```python
from build123d import *

# Parameters (mm, degrees)
SKETCH1_W           = 23
SKETCH1_H           = 13
BOSS_EXTRUDE1_DEPTH = 18
SKETCH2_W           = 33
SKETCH2_H           = 13
BOSS_EXTRUDE2_DEPTH = 2.5
SKETCH3_W           = 23
SKETCH3_H           = 13
BOSS_EXTRUDE3_DEPTH = 1.5
BOSS_EXTRUDE4_DEPTH = 5.5
SKETCH5_R           = 2.4
BOSS_EXTRUDE5_DEPTH = 4


with BuildPart() as part:
    # Sketch1 → Boss-Extrude1 (new body)
    with BuildSketch(Plane(origin=(0, 0, 0), x_dir=(1, 0, 0), z_dir=(0, 1, 0))):
        Rectangle(SKETCH1_W, SKETCH1_H)
    extrude(amount=BOSS_EXTRUDE1_DEPTH)

    # Sketch2 → Boss-Extrude2 (add)
    with BuildSketch(Plane(origin=(0, 18, 0), x_dir=(1, 0, 0), z_dir=(0, 1, 0))):
        Rectangle(SKETCH2_W, SKETCH2_H)
    extrude(amount=BOSS_EXTRUDE2_DEPTH)

    # Sketch3 → Boss-Extrude3 (add)
    with BuildSketch(Plane(origin=(0, 20.5, 0), x_dir=(1, 0, 0), z_dir=(0, 1, 0))):
        Rectangle(SKETCH3_W, SKETCH3_H)
    extrude(amount=BOSS_EXTRUDE3_DEPTH)

    # Sketch4 → Boss-Extrude4 (add)
    with BuildSketch(Plane(origin=(0, 22, 0), x_dir=(1, 0, 0), z_dir=(0, 1, 0))):
        with BuildLine():
            ThreePointArc((0.918269231, 2.687766603), (-11.5, 0), (0.918269231, -2.687766603))
            ThreePointArc((0.918269231, -2.687766603), (4.25, 0), (0.918269231, 2.687766603))
        make_face()
    extrude(amount=BOSS_EXTRUDE4_DEPTH)

    # Sketch5 → Boss-Extrude5 (add)
    with BuildSketch(Plane(origin=(0, 27.5, 0), x_dir=(1, 0, 0), z_dir=(0, 1, 0))):
        with Locations(Location((-5, 0, 0), (0, 0, 270))):
            Circle(SKETCH5_R)
    extrude(amount=BOSS_EXTRUDE5_DEPTH)


solid = part.part
```
Verification items for the finished model (mm, model axes). A direction names the side the tool comes from. Coordinates: 2 decimals unless noted, no trailing zeros. Loops run counter-clockwise (first coordinate to the right, second up) from the corner with the lowest first, then second, coordinate; pieces in that order, holes last. Notation, with made-up numbers: (34.5, 57) - (51.5, 57) arc R15 ccw to (51.5, 72) - close; hole circle Ø11 at (63, 60). An arc over 180 degrees is marked (long way). Put each result on its own line as item: value.
Item 1: Section check D-D (x = 14). Enter the section's corners in (y, z).
Conclusion:
outline: (18, -6.5) - (20.5, -6.5) - (20.5, 6.5) - (18, 6.5) - close
Item 2: Section check B-B (z = -4.5). Enter the section's corners in (x, y), then the cut area to 3 significant figures.
Conclusion:
outline: (-16.5, 18) - (-11.5, 18) - (-11.5, 0) - (11.5, 0) - (11.5, 18) - (16.5, 18) - (16.5, 20.5) - (11.5, 20.5) - (11.5, 22) - (-0.31, 22) - (-0.31, 27.5) - (-9.69, 27.5) - (-9.69, 22) - (-11.5, 22) - (-11.5, 20.5) - (-16.5, 20.5) - close
area: 583 mm2
Item 3: Set-up check for faces 1 (the face through (11.5, 21, 0)), 2 (the face through (14, 18, 0)), 3 (the face through (-2.976, 29.472, 1.29)): record each of +Z, -Z, +X, -X, +Y, -Y from which the full face is reachable in a straight line by a thin tool's end or side.
Conclusion:
face 1: +Z, -Z, +X, +Y
face 2: +Z, -Z, +X, -Y
face 3: +Y
Item 4: Gauge pin test, flat ends, axial feed: pin 1 Ø1.5 at (x, z) = (5, 4.5) entering from -Y; pin 2 Ø2 at (x, z) = (8.5, 1.5) entering from +Y; pin 3 Ø1.5 at (x, z) = (13.5, -1.5) entering from -Y; pin 4 Ø2.5 at (x, z) = (-15, 2) entering from +Y. Record the tip position at first contact, or that the pin passes through.
Conclusion:
pin 1: stops at y = 0
pin 2: stops at y = 22
pin 3: stops at y = 18
pin 4: stops at y = 20.5
Item 5: Section check C-C (y = 16.5). Enter the section's corners in (x, z).
Conclusion:
outline: (-11.5, -6.5) - (11.5, -6.5) - (11.5, 6.5) - (-11.5, 6.5) - close
Item 6: Section check A-A (x = 1.5). Enter the section's corners in (y, z).
Conclusion:
outline: (0, -6.5) - (22, -6.5) - (22, -2.75) - (27.5, -2.75) - (27.5, 2.75) - (22, 2.75) - (22, 6.5) - (0, 6.5) - close
Item 7: Scan lines: line 1 along X through (y, z) = (4, -3); line 2 along Y through (x, z) = (12, -5.75); line 3 along Y through (x, z) = (-1.5, 0). Record each from-to range of solid material in increasing order.
Conclusion:
line 1: x = -11.5 to 11.5
line 2: y = 18 to 20.5
line 3: y = 0 to 27.5
